Source: CAD feature listing. Evaluate the final solid. Frame: model axes, mm. A direction names the side the tool comes from. Coordinates: 2 decimals unless noted, no trailing zeros. Loops run counter-clockwise (first coordinate to the right, second up) from the corner with the lowest first, then second, coordinate; pieces in that order, holes last. Notation, with made-up numbers: (17, -7.75) - (34, -7.75) arc R29 ccw to (34, 17.25) - close; hole circle Ø7 at (4.25, 70.25). An arc over 180 degrees is marked (long way). Use CSV: the item, a comma, the result in double quotes. Start each with the question number.
```python
from build123d import *

# Parameters (mm, degrees)
SKETCH_1_W          = 216
SKETCH_1_H          = 114
EXTRUDE_1_DEPTH     = 50
SKETCH_2_W          = 27.595124593
SKETCH_2_H          = 108.683413436
CUT_EXTRUDE_1_DEPTH = 44
SKETCH_3_W          = 15.377269527
SKETCH_3_H          = 95.391197403
EXTRUDE_2_DEPTH     = 10
SKETCH_4_R          = 1.5
CUT_EXTRUDE_2_DEPTH = 115


with BuildPart() as part:
    # 草图1 → 凸台-拉伸1 (new body)
    with BuildSketch(Plane(origin=(0, 0, 0), x_dir=(1, 0, 0), z_dir=(0, 1, 0))):
        Rectangle(SKETCH_1_W, SKETCH_1_H)
    extrude(amount=EXTRUDE_1_DEPTH)

    # 草图2 → 切除-拉伸1 (cut)
    with BuildSketch(Plane(origin=(0, 50, 0), x_dir=(1, 0, 0), z_dir=(0, 1, 0))):
        with Locations((-94.202437704, 0)):
            Rectangle(SKETCH_2_W, SKETCH_2_H)
    extrude(amount=-CUT_EXTRUDE_1_DEPTH, mode=Mode.SUBTRACT)

    # 草图3 → 凸台-拉伸2 (add)
    with BuildSketch(Plane(origin=(0, 6, 0), x_dir=(1, 0, 0), z_dir=(0, 1, 0))):
        with Locations((-94.609302344, 0.130315844)):
            Rectangle(SKETCH_3_W, SKETCH_3_H)
    extrude(amount=EXTRUDE_2_DEPTH)

    # 草图4 → 切除-拉伸2 (cut, through all)
    with BuildSketch(Plane.XY.offset(57)):
        with Locations((75.5, 37.5)):
            Circle(SKETCH_4_R)
        with Locations((75.5, 12.5)):
            Circle(SKETCH_4_R)
        with Locations((-75.5, 12.5)):
            Circle(SKETCH_4_R)
        with Locations((-75.5, 37.5)):
            Circle(SKETCH_4_R)
    extrude(amount=-CUT_EXTRUDE_2_DEPTH, mode=Mode.SUBTRACT)


solid = part.part
```
(1) Pin query (flat end, axial travel): pin 1 Ø1.5 at (x, z) = (-82, 21) entering from +Y; pin 2 Ø22 at (y, z) = (32, 25.5) entering from -X; pin 3 Ø2 at (y, z) = (12.5, 28) entering from -X. Return the tip coordinate at first contact, or that it passes through.
(2) Ray query, line 1 (Z direction, x = -97, y = 12); line 2 (Y direction, x = 75.5, z = 17); line 3 (Y direction, x = -75, z = -10). Return the intervals inside material, ascending. Write a range as [from, to].
(3) Section A-A on z = -6.5. Output: boundary loops of the cut face in (x, y), plus the area to 3 significant figures.
(4) Reachability of faces 4 (the flat face through (-80.405, 28, 1)), 5 (the flat face through (-102.298, 11, 1)), 6 (the flat face through (-2, 25, 57)) from +Z, -Z, +X, -X, +Y, -Y: full face, straight path, thin tool, end or side. Return the list, or none.
(5) Section C-C on y = 22. Output: boundary loops of the cut face in (x, z).
(6) Section B-B on y = 9. Output: boundary loops of the cut face in (x, z).
(7) Draft query along X for faces 1 (the flat face through (108, 25, 1)), 2 (the flat face through (-2, 50, -1)), 3 (the flat face through (-86.921, 11, 1)). Return one class per face: released by +X, released by -X, zero draft, split by the parting line, or undercut.
Solution:
1,pin 1,"stops at y = 6"
1,pin 2,"stops at x = -80.4"
1,pin 3,"stops at x = -102.3"
2,line 1,"z = [-57, -54.34], [-47.83, 47.57], [54.34, 57]"
2,line 2,"y = [0, 11], [14, 36], [39, 50]"
2,line 3,"y = [0, 11.09], [13.91, 36.09], [38.91, 50]"
3,outline,"(-108, 0) - (108, 0) - (108, 50) - (-80.4, 50) - (-80.4, 6) - (-86.92, 6) - (-86.92, 16) - (-102.3, 16) - (-102.3, 6) - (-108, 6) - close; hole circle Ø3 at (-75.5, 12.5); hole circle Ø3 at (-75.5, 37.5); hole circle Ø3 at (75.5, 12.5); hole circle Ø3 at (75.5, 37.5)"
3,area,"9,710 mm²"
4,face 4,"+Y"
4,face 5,"-X, +Y"
4,face 6,"+Z, +X, -X, +Y, -Y"
5,outline,"(-108, -57) - (108, -57) - (108, 57) - (-108, 57) - (-108, 54.34) - (-80.4, 54.34) - (-80.4, -54.34) - (-108, -54.34) - close"
6,outline,"(-108, -57) - (108, -57) - (108, 57) - (-108, 57) - (-108, 54.34) - (-80.4, 54.34) - (-80.4, -54.34) - (-108, -54.34) - close; (-102.3, -47.83) - (-86.92, -47.83) - (-86.92, 47.57) - (-102.3, 47.57) - close"
7,face 1,"released by +X"
7,face 2,"zero draft"
7,face 3,"undercut"
